Model file for the job. Use its own axes, mm. A direction names the side the tool comes from. Round coordinates to 2 decimals unless told otherwise and drop trailing zeros. Order: outer loops, then holes, each group sorted by start corner. A loop starts at its lowest first (then second) coordinate and runs counter-clockwise, first axis right, second up. Notation, with made-up numbers: (41.5, -6) - (63.5, -6) arc R17 cw to (63.5, 1) - close; hole circle Ø1 at (60, 61). An arc over 180 degrees is marked (long way). Write item = value, one per line.
```python
from build123d import *

# Parameters (mm, degrees)
SKETCH2_R               = 7.5
BOSS_EXTRUDE1_DEPTH     = 24
CUT_EXTRUDE2_DEPTH      = 40.913473307
CUT_EXTRUDE2_DEPTH_BACK = 40.913473307
SKETCH5_W               = 68.617197106
SKETCH5_H               = 1
SKETCH6_W               = 14.2
SKETCH6_H               = 9
CUT_EXTRUDE4_DEPTH      = 40.913473307
SKETCH7_R               = 1.5
CUT_EXTRUDE5_DEPTH      = 7
CUT_EXTRUDE6_DEPTH      = 40.913473307
CUT_EXTRUDE6_DEPTH_BACK = 40.913473307
SKETCH9_W               = 33.569510153
SKETCH9_H               = 1
CUT_EXTRUDE7_DEPTH      = 10
CUT_EXTRUDE8_DEPTH      = 42.952353927
CUT_EXTRUDE8_DEPTH_BACK = 6


with BuildPart() as part:
    # Sketch2 → Boss-Extrude1 (new body)
    with BuildSketch(Plane.XY):
        with BuildLine():
            Line((-17.5, -5.732866955), (-5, -5.732866955))
            Line((-5, -5.732866955), (17.5, -5.732866955))
            ThreePointArc((17.5, -5.732866955), (28, 4.767133045), (17.5, 15.267133045))
            Line((17.5, 15.267133045), (-17.5, 15.267133045))
            ThreePointArc((-17.5, 15.267133045), (-28, 4.767133045), (-17.5, -5.732866955))
        make_face()
        with Locations((-17.5, 4.767133045)):
            Circle(SKETCH2_R, mode=Mode.SUBTRACT)
        with Locations((17.5, 4.767133045)):
            Circle(SKETCH2_R, mode=Mode.SUBTRACT)
    extrude(amount=BOSS_EXTRUDE1_DEPTH)

    # Sketch5 → Cut-Extrude2 (cut, two sides: drawn at the far end of the back side and taken through both)
    with BuildSketch(Plane(origin=(0, 0, 0), x_dir=(-1, 0, 0), z_dir=(0, 0, -1)).offset(-CUT_EXTRUDE2_DEPTH_BACK)):
        with Locations((-5.849443293, -5.232866955)):
            Rectangle(SKETCH5_W, SKETCH5_H)
    extrude(amount=CUT_EXTRUDE2_DEPTH + CUT_EXTRUDE2_DEPTH_BACK, mode=Mode.SUBTRACT)

    # Sketch6 → Cut-Extrude4 (cut, through all)
    with BuildSketch(Plane(origin=(0, 0, 0), x_dir=(-1, 0, 0), z_dir=(0, 0, -1))):
        with Locations((0, 7.567133045)):
            Rectangle(SKETCH6_W, SKETCH6_H)
    extrude(amount=-CUT_EXTRUDE4_DEPTH, mode=Mode.SUBTRACT)

    # Sketch7 → Cut-Extrude5 (cut)
    with BuildSketch(Plane(origin=(0, 15.267133045, 0), x_dir=(1, 0, 0), z_dir=(0, 1, 0))):
        with Locations(Location((0, -5, 0), (0, 0, 270))):
            Circle(SKETCH7_R)
        with Locations(Location((0, -17, 0), (0, 0, 270))):
            Circle(SKETCH7_R)
    extrude(amount=-CUT_EXTRUDE5_DEPTH, mode=Mode.SUBTRACT)

    # Sketch8 → Cut-Extrude6 (cut, two sides: drawn at the far end of the back side and taken through both)
    with BuildSketch(Plane(origin=(0, 0, 0), x_dir=(0, 0, -1), z_dir=(1, 0, 0)).offset(-CUT_EXTRUDE6_DEPTH_BACK)):
        Polygon((-26.475275498, 0), (-18.93282628, -6.456635217), (-28.387151922, -5.921555858), align=None)
    extrude(amount=CUT_EXTRUDE6_DEPTH + CUT_EXTRUDE6_DEPTH_BACK, mode=Mode.SUBTRACT)

    # Sketch9 → Cut-Extrude7 (cut)
    with BuildSketch(Plane(origin=(30, 0, 0), x_dir=(0, 0, -1), z_dir=(1, 0, 0))):
        with Locations((-12.766874728, 5.267133045)):
            Rectangle(SKETCH9_W, SKETCH9_H)
    cut_extrude7 = extrude(amount=-CUT_EXTRUDE7_DEPTH, mode=Mode.SUBTRACT)

    # Mirror1: Cut-Extrude7 across plane
    add(cut_extrude7.mirror(Plane(origin=(0, 0, 0), x_dir=(0, 0, 1), z_dir=(1, 0, 0))), mode=Mode.SUBTRACT)

    # Sketch11 → Cut-Extrude8 (cut, two sides: drawn at the far end of the back side and taken through both)
    with BuildSketch(Plane(origin=(0, 15.267133045, 0), x_dir=(1, 0, 0), z_dir=(0, 1, 0)).offset(-CUT_EXTRUDE8_DEPTH_BACK)):
        with BuildLine():
            Line((-1.5, -18.944592398), (-1.5, -15.189153247))
            ThreePointArc((-1.5, -15.189153247), (0, -13.689153247), (1.5, -15.189153247))
            Line((1.5, -15.189153247), (1.5, -18.944592398))
            ThreePointArc((1.5, -18.944592398), (0, -20.444592398), (-1.5, -18.944592398))
        make_face()
        with BuildLine():
            Line((-1.492419394, -7.149757539), (-1.492419394, -3.394318388))
            ThreePointArc((-1.492419394, -3.394318388), (0.007580606, -1.894318388), (1.507580606, -3.394318388))
            Line((1.507580606, -3.394318388), (1.507580606, -7.149757539))
            ThreePointArc((1.507580606, -7.149757539), (0.007580606, -8.649757539), (-1.492419394, -7.149757539))
        make_face()
    extrude(amount=CUT_EXTRUDE8_DEPTH + CUT_EXTRUDE8_DEPTH_BACK, mode=Mode.SUBTRACT)


solid = part.part
```
1) Cut at C-C (y = 8). Write the cut outline in (x, z), and give its area (3 significant figures).
Conclusion:
outline = (-27.49, 0) - (-24.27, 0) - (-24.27, 24) - (-27.49, 24) - close; (-10.73, 0) - (-7.1, 0) - (-7.1, 24) - (-10.73, 24) - close; (7.1, 0) - (10.73, 0) - (10.73, 24) - (7.1, 24) - close; (24.27, 0) - (27.49, 0) - (27.49, 24) - (24.27, 24) - close
area = 329 mm^2
2) Mould opens along Z. For faces 4 (the face through (25, 1, 24)), 5 (the face through (26.32, -0.93, 11.83)), 6 (the face through (-1.5, 14, 17)) say: +Z half, -Z half, draft (parallel to the pull), parting line (faces both ways), or undercut.
Conclusion:
face_4 = +Z half
face_5 = draft
face_6 = undercut
3) 3-axis set-ups, long thin cutter, end or side, ignore diameter. For faces 1 (the face through (-26, 5.767, 12)), 2 (the face through (0, 12.067, 12)), 3 (the face through (1.5, 14, 17)): which of +Z, -Z, +X, -X, +Y, -Y reach the whole face in a straight line?
Conclusion:
face_1 = +Z, -Z, -X
face_2 = +Z, -Z
face_3 = +Y
4) Flat gauge pins, fed straight in: pin 1 Ø3.5 at (y, z) = (13.5, 17.5) entering from -X; pin 2 Ø0.7 at (y, z) = (14, 4) entering from +X; pin 3 Ø7 at (y, z) = (9.5, 7) entering from -X. Where does each tip first touch, or does it go through?
Conclusion:
pin_1 = -25.34
pin_2 = 23.1
pin_3 = -27.93
5) Wall check: line 1 along Y through (x, z) = (-2, 20.5); line 2 along Y through (x, z) = (-17.5, 7); line 3 along X through (y, z) = (11.5, 9.5). Give the ranges that are in metal, low to high.
Conclusion:
line_1 = -4.73 to 3.07, 12.07 to 15.27
line_2 = -4.73 to -2.73, 12.27 to 15.27
line_3 = -25.56 to -20.8, -14.2 to -7.1, 7.1 to 14.2, 20.8 to 25.56
6) Cut at D-D (x = 0). Write the cut outline in (y, z), and give its area (3 significant figures).
Conclusion:
outline = (-4.73, 0) - (3.07, 0) - (3.07, 24) - (-2.12, 24) - (-4.73, 20.95) - close; (12.07, 0) - (15.27, 0) - (15.27, 1.89) - (12.07, 1.89) - close; (12.07, 8.65) - (15.27, 8.65) - (15.27, 13.69) - (12.07, 13.69) - close; (12.07, 20.44) - (15.27, 20.44) - (15.27, 24) - (12.07, 24) - close
area = 217 mm^2
7) Cut at A-A (x = -13). Write the cut outline in (y, z), and give its area (3 significant figures).
Conclusion:
outline = (-4.73, 0) - (-1.23, 0) - (-1.23, 24) - (-2.12, 24) - (-4.73, 20.95) - close; (10.77, 0) - (15.27, 0) - (15.27, 24) - (10.77, 24) - close
area = 188 mm^2
8) Cut at B-B (z = 16.25). Write the cut outline in (x, y), and give its area (3 significant figures).
Conclusion:
outline = (-28, 4.77) arc R10.5 ccw to (-21.97, -4.73) - (21.97, -4.73) arc R10.5 ccw to (28, 4.77) - (25, 4.77) arc R7.5 cw (long way) to (24.93, 5.77) - (27.95, 5.77) arc R10.5 ccw to (17.5, 15.27) - (1.5, 15.27) - (1.5, 12.07) - (7.1, 12.07) - (7.1, 3.07) - (-7.1, 3.07) - (-7.1, 12.07) - (-1.5, 12.07) - (-1.5, 15.27) - (-17.5, 15.27) arc R10.5 ccw to (-27.95, 5.77) - (-24.93, 5.77) arc R7.5 cw (long way) to (-25, 4.77) - close
area = 543 mm^2
